from build123d import *

# Parameters (mm, degrees)
SKETCH1_R           = 35.65
SKETCH1_W           = 3.8
SKETCH1_H           = 39.7
BOSS_EXTRUDE1_DEPTH = 4
FILLET1_R           = 10.5


with BuildPart() as part:
    # Sketch1 → Boss-Extrude1 (new body)
    with BuildSketch(Plane(origin=(0, 0, 0), x_dir=(1, 0, 0), z_dir=(0, 1, 0))):
        with Locations(Location((0, 0, 0), (0, 0, 270))):
            Circle(SKETCH1_R)
        with BuildLine():
            Line((4.3, -31.053703483), (4.3, 31.053703483))
            ThreePointArc((4.3, 31.053703483), (31.35, 0), (4.3, -31.053703483))
        make_face(mode=Mode.SUBTRACT)
        with BuildLine():
            Line((-4.3, -31.053703483), (-4.3, 31.053703483))
            ThreePointArc((-4.3, 31.053703483), (-31.35, 0), (-4.3, -31.053703483))
        make_face(mode=Mode.SUBTRACT)
        Rectangle(SKETCH1_W, SKETCH1_H, mode=Mode.SUBTRACT)
    extrude(amount=BOSS_EXTRUDE1_DEPTH)

    # Fillet1
    fillet1_edges = [part.edges().sort_by_distance(p)[0] for p in [
        (4.3, 2, -31.053703483),
        (4.3, 2, 31.053703483),
        (-4.3, 2, 31.053703483),
        (-4.3, 2, -31.053703483),
    ]]
    fillet(fillet1_edges, radius=FILLET1_R)


solid = part.part
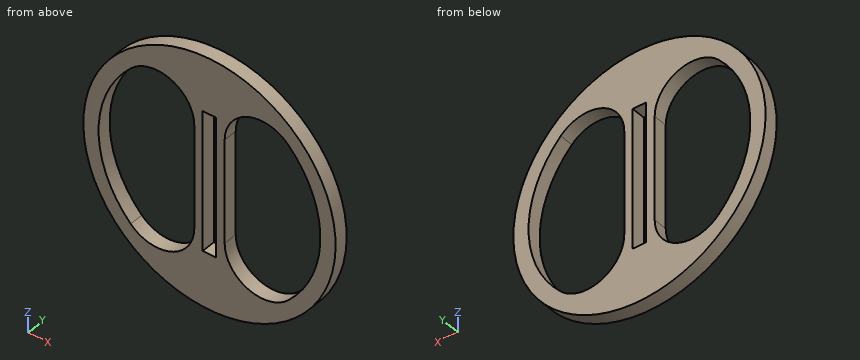
Model file for the job. Use its own axes, mm. Coordinates: 2 decimals unless noted, no trailing zeros. Order: outer loops, then holes, each group sorted by start corner. A loop starts at its lowest first (then second) coordinate and runs counter-clockwise, first axis right, second up. Notation, with made-up numbers: M -17.75,60 L -11.75,60 A37 ccw -11.75,96 Z; hole C -4,64 d6. An arc over 180 degrees is marked long. Return JSON: item names as keys, results as strings.
1. Saw through at A-A (x = 0). Give the cut face in (y, z), and give its area (3 significant figures).
Ans:
{"outline": "M 0,-35.65 L 4,-35.65 L 4,-19.85 L 0,-19.85 Z; M 0,19.85 L 4,19.85 L 4,35.65 L 0,35.65 Z", "area": "126 mm^2"}
2. Flat gauge pins, fed straight in: pin 1 (1.2 mm diameter, centred on y = 1, z = 0.5, fed in from -X); pin 2 (1.2 mm diameter, centred on y = 1.5, z = -4.5, fed in from +X). Where does each tip first touch, or does it go through?
Ans:
{"pin 1": "x = -35.65", "pin 2": "x = 35.44"}
3. Saw through at C-C (y = 1.2). Give the cut face in (x, z).
Ans:
{"outline": "C 0,0 d71.3; hole M -22.25,-22.08 A10.5 ccw -4.3,-14.69 L -4.3,14.69 A10.5 ccw -22.25,22.08 A31.35 ccw Z; hole M -1.9,-19.85 L 1.9,-19.85 L 1.9,19.85 L -1.9,19.85 Z; hole M 4.3,-14.69 A10.5 ccw 22.25,-22.08 A31.35 ccw 22.25,22.08 A10.5 ccw 4.3,14.69 Z"}
4. Saw through at D-D (z = -13). Give the cut face in (x, y), and give its area (3 significant figures).
Ans:
{"outline": "M -33.2,0 L -28.53,0 L -28.53,4 L -33.2,4 Z; M -4.3,0 L -1.9,0 L -1.9,4 L -4.3,4 Z; M 1.9,0 L 4.3,0 L 4.3,4 L 1.9,4 Z; M 28.53,0 L 33.2,0 L 33.2,4 L 28.53,4 Z", "area": "56.5 mm^2"}
5. Saw through at B-B (z = 0). Give the cut face in (x, y), and give its area (3 significant figures).
Ans:
{"outline": "M -35.65,0 L -31.35,0 L -31.35,4 L -35.65,4 Z; M -4.3,0 L -1.9,0 L -1.9,4 L -4.3,4 Z; M 1.9,0 L 4.3,0 L 4.3,4 L 1.9,4 Z; M 31.35,0 L 35.65,0 L 35.65,4 L 31.35,4 Z", "area": "53.6 mm^2"}
6. Drill centre lines: probe 1 along X at (y, z) = (1.7, 17); probe 2 along X at (y, z) = (2.1, -14.5); probe 3 along X at (y, z) = (2.3, 21.5). Where is each one in solid material? Low to high.
Ans:
{"probe 1": "-31.34 to -26.34, -4.56 to -1.9, 1.9 to 4.56, 26.34 to 31.34", "probe 2": "-32.57 to -27.8, -4.3 to -1.9, 1.9 to 4.3, 27.8 to 32.57", "probe 3": "-28.44 to -22.82, -6.81 to 6.81, 22.82 to 28.44"}
